Here's the drawing with two shaded views (mm, measured from the low corner). I have some questions. Coordinates: 2 decimals unless noted, no trailing zeros. Write each loop counter-clockwise with the first axis right and the second up, starting at its lowest first coordinate (ties: lowest second). Pieces come first, ordered by that corner, then holes. Notation, with made-up numbers: (15.25, 76) -> (61.25, 76) arc R28 cw to (61.25, 106) -> close; hole circle Ø1 at (0.5, 23.25). An arc over 180 degrees is marked (long way). Use a Markdown table: item, result. Add a question column.
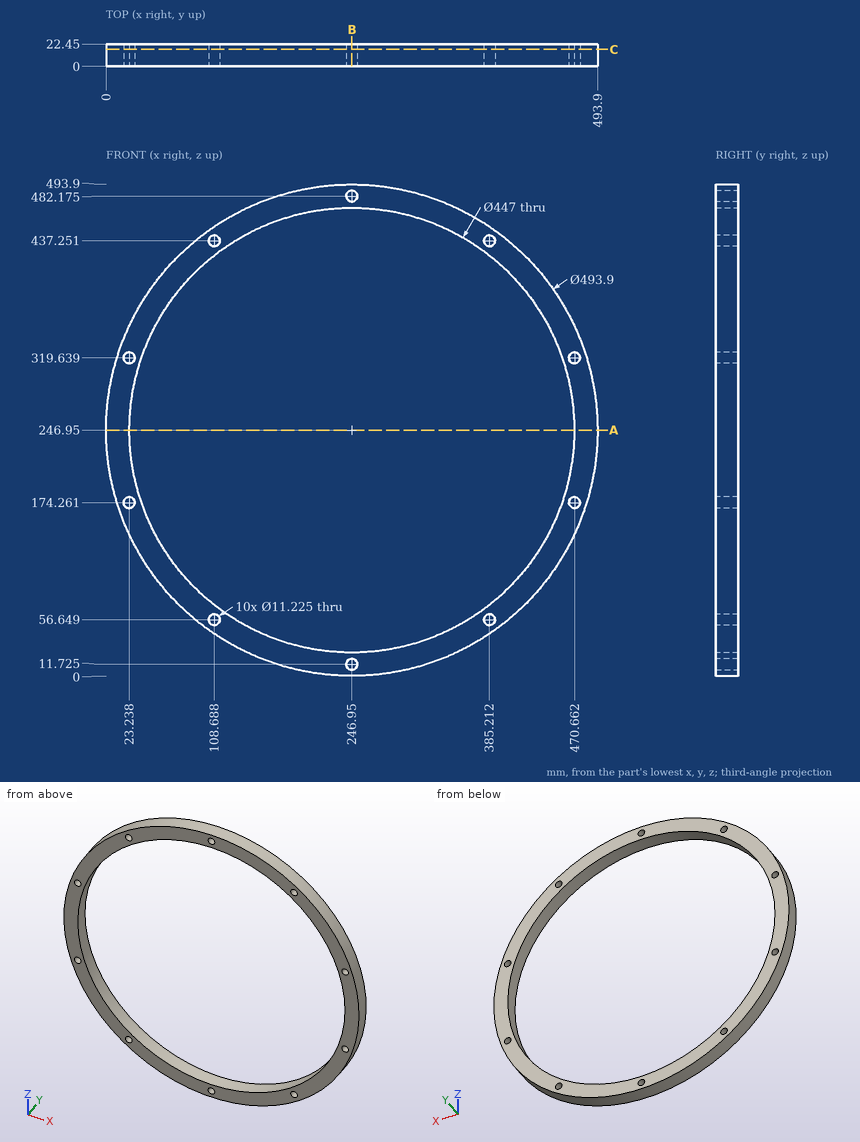
Q1. Suppose I cut it at C-C, the plane y = 17. State how many separate pieces and enclosed holes the cut face has, and give its area (3 significant figures).
Q2. Please list where these lines run through material, in increasing order: line 1 (X direction, y = 14.5, z = 60) (1 decimal); line 2 (X direction, y = 4.75, z = 392) (1 decimal); line 3 (X direction, y = 3.5, z = 361) (1 decimal).
Q3. Suppose I cut it at B-B, the plane x = 246.95. Write out the boundary of the cut face in (y, z), and give its area (3 significant figures).
Q4. Will these pins go through, and if not, where does the flat tip stop? pin 1 (1 mm diameter, centred on x = 76.5, y = 6.5, fed in from +Z); pin 2 (10 mm diameter, centred on y = 19.5, z = 406.5, fed in from +X); pin 3 (12 mm diameter, centred on y = 6.5, z = 238, fed in from -X).
Q5. Suppose I cut it at A-A, the plane z = 246.95. Write out the boundary of the cut face in (x, y), and give its area (3 significant figures).
Answer key:
| question | item | result |
|---|---|---|
| 1 | separate pieces | 1 |
| 1 | enclosed holes | 11 |
| 1 | area | 33,700 mm^2 |
| 2 | line 1 | x = 85.6 to 104.2, 113.2 to 124.5, 369.4 to 380.7, 389.7 to 408.3 |
| 2 | line 2 | x = 47.1 to 76.9, 417 to 446.8 |
| 2 | line 3 | x = 27.9 to 54.7, 439.2 to 466 |
| 3 | outline | (0, 0) -> (22.45, 0) -> (22.45, 6.11) -> (0, 6.11) -> close; (0, 17.34) -> (22.45, 17.34) -> (22.45, 23.45) -> (0, 23.45) -> close; (0, 470.45) -> (22.45, 470.45) -> (22.45, 476.56) -> (0, 476.56) -> close; (0, 487.79) -> (22.45, 487.79) -> (22.45, 493.9) -> (0, 493.9) -> close |
| 3 | area | 549 mm^2 |
| 4 | pin 1 | stops at z = 426.12 |
| 4 | pin 2 | stops at x = 439.56 |
| 4 | pin 3 | stops at x = 0.02 |
| 5 | outline | (0, 0) -> (23.45, 0) -> (23.45, 22.45) -> (0, 22.45) -> close; (470.45, 0) -> (493.9, 0) -> (493.9, 22.45) -> (470.45, 22.45) -> close |
| 5 | area | 1,050 mm^2 |
